```python
from build123d import *

# Parameters (mm, degrees)
F0_W     = 60
F0_H     = 40
F1_DEPTH = 1.6
F2_W     = 0.8
F2_H     = 40
F2_W_2   = 1.2
F2_W_3   = 1.6
F2_W_4   = 2
F2_W_5   = 2.4
F2_W_6   = 3
F2_W_7   = 3.4
F2_W_8   = 20
F2_H_2   = 0.8
F2_H_3   = 1.2
F2_H_4   = 1.6
F2_H_5   = 2
F3_DEPTH = 15


with BuildPart() as f1:
    # F0 (on Top) → F1 (new body)
    with BuildSketch(Plane.XY):
        with Locations((30, -20)):
            Rectangle(F0_W, F0_H)
    extrude(amount=F1_DEPTH)

    # F2 (on face) → F3 (join)
    with BuildSketch(Plane.XY.offset(1.6)):
        with Locations((5.4, -20)):
            Rectangle(F2_W, F2_H)
        with Locations((7.6, -20)):
            Rectangle(F2_W_2, F2_H)
        with Locations((10.6, -20)):
            Rectangle(F2_W_3, F2_H)
        with Locations((14.4, -20)):
            Rectangle(F2_W_4, F2_H)
        with Locations((19, -20)):
            Rectangle(F2_W_5, F2_H)
        with Locations((24.7, -20)):
            Rectangle(F2_W_6, F2_H)
        with Locations((31.3, -20)):
            Rectangle(F2_W_7, F2_H)
        with Locations((50, -29.2)):
            Rectangle(F2_W_8, F2_H_2)
        with Locations((50, -20.2)):
            Rectangle(F2_W_8, F2_H_3)
        with Locations((50, -10.8)):
            Rectangle(F2_W_8, F2_H_4)
        with Locations((50, -1)):
            Rectangle(F2_W_8, F2_H_5)
    extrude(amount=F3_DEPTH)


solid = f1.part
```
Source: CAD feature listing. Evaluate the final solid. Frame: model axes, mm. A direction names the side the tool comes from. Round coordinates to 2 decimals unless told otherwise and drop trailing zeros. Loops run counter-clockwise (first coordinate to the right, second up) from the corner with the lowest first, then second, coordinate; pieces in that order, holes last. Notation, with made-up numbers: M 50.25,-20 L 71.25,-20 A19 ccw 71.25,-15 Z; hole C -2,85.25 d11. An arc over 180 degrees is marked long. Use a Markdown table: item, result. Add a question column.
1. Cut plane B-B, the plane x = 49.5. Output: boundary loops of the cut face in (y, z), and give its area (3 significant figures).
2. Cut plane D-D, the plane x = 12.5. Output: boundary loops of the cut face in (y, z).
3. Set-up query: faces 1 (the flat face through (15.4, -20, 9)), 2 (the flat face through (50, -11.6, 9)), 3 (the flat face through (5, -20, 9)). Return all of +Z, -Z, +X, -X, +Y, -Y with unobstructed straight access to the full face (end or side cutting, diameter ignored); none if empty.
4. Ray query, line 1 along Y through (x, z) = (41.5, 4.75); line 2 along Z through (x, y) = (52, -12). Return the intervals inside material, ascending. Write a range as [from, to].
5. Contact query for flat-ended pins moving along their axis: pin 1 (0.8 mm diameter, centred on y = -10.5, z = 9.5, fed in from -X); pin 2 (2.5 mm diameter, centred on x = 2.5, y = -21, fed in from +Z); pin 3 (4 mm diameter, centred on y = -35.5, z = 10.5, fed in from +X). Output: stop coordinate, or through.
6. Cut plane C-C, the plane z = 12. State how many separate pieces and enclosed holes the cut face has, and give its area (3 significant figures).
7. Pull-direction query (Y, two-part tool) for faces 4 (the flat face through (46, -24, 1.6)), 5 (the flat face through (5.8, -20, 9)), 6 (the flat face through (50, -20.8, 9)); classes: +Y half, -Y half, draft (parallel to the pull), parting line (faces both ways), or undercut.
Solution:
| question | item | result |
|---|---|---|
| 1 | outline | M -40,0 L 0,0 L 0,16.6 L -2,16.6 L -2,1.6 L -10,1.6 L -10,16.6 L -11.6,16.6 L -11.6,1.6 L -19.6,1.6 L -19.6,16.6 L -20.8,16.6 L -20.8,1.6 L -28.8,1.6 L -28.8,16.6 L -29.6,16.6 L -29.6,1.6 L -40,1.6 Z |
| 1 | area | 148 mm2 |
| 2 | outline | M -40,0 L 0,0 L 0,1.6 L -40,1.6 Z |
| 3 | face 1 | +Z, +Y, -Y |
| 3 | face 2 | +Z, +X |
| 3 | face 3 | +Z, -X, +Y, -Y |
| 4 | line 1 | y = [-29.6, -28.8], [-20.8, -19.6], [-11.6, -10], [-2, 0] |
| 4 | line 2 | z = [0, 1.6] |
| 5 | pin 1 | stops at x = 5 |
| 5 | pin 2 | stops at z = 1.6 |
| 5 | pin 3 | stops at x = 33 |
| 6 | separate pieces | 11 |
| 6 | enclosed holes | 0 |
| 6 | area | 688 mm2 |
| 7 | face 4 | undercut |
| 7 | face 5 | draft |
| 7 | face 6 | undercut |
